The model under review builds one solid part; all positions refer to its coordinate system, in mm. A direction names the side the tool comes from. Round coordinates to 2 decimals unless told otherwise and drop trailing zeros. Order: outer loops, then holes, each group sorted by start corner. A loop starts at its lowest first (then second) coordinate and runs counter-clockwise, first axis right, second up. Notation, with made-up numbers: (-39, 2.25) -> (-30, 2.25) arc R29 cw to (-30, 37.25) -> close; hole circle Ø5 at (82.25, 25). An arc over 180 degrees is marked (long way). Use a Markdown table: item, result. Add a question column.
```python
from build123d import *

# Parameters (mm, degrees)
SKETCH1_W           = 70
SKETCH1_H           = 12
BOSS_EXTRUDE1_DEPTH = 1.5
SKETCH2_W           = 60
SKETCH2_H           = 6
CUT_EXTRUDE1_DEPTH  = 38.121422387
FILLET1_R           = 10
FILLET2_R           = 5
SKETCH3_W           = 3
SKETCH3_H           = 4
BOSS_EXTRUDE2_DEPTH = 3


with BuildPart() as part:
    # Sketch1 → Boss-Extrude1 (new, symmetric)
    with BuildSketch(Plane.XY):
        with Locations((0, 6)):
            Rectangle(SKETCH1_W, SKETCH1_H)
    extrude(amount=BOSS_EXTRUDE1_DEPTH, both=True)

    # Sketch2 → Cut-Extrude1 (cut, through all)
    with BuildSketch(Plane.XY.offset(1.5)):
        with Locations((0, 9)):
            Rectangle(SKETCH2_W, SKETCH2_H)
    extrude(amount=-CUT_EXTRUDE1_DEPTH, mode=Mode.SUBTRACT)

    # Fillet1
    # the kernel refuses this fillet: 10 mm, written as the material it adds along each edge
    with BuildSketch(Plane(origin=(30, 6, 1.5), x_dir=(-1, 0, 0), z_dir=(0, 0, -1))) as fillet1_piece_1:
        with BuildLine():
            CenterArc((9.16515139, 10), FILLET1_R, 203.578178478, 66.421821522)
            Line((0, 6), (-0.183303028, 5.92))
            ThreePointArc((-0.183303028, 5.92), (-0.2, 3), (-0.2, 0))
            Line((-0.2, 0), (0, -0.2))
            Line((0, -0.2), (9.16515139, -0.2))
            Line((9.16515139, -0.2), (9.16515139, 0))
        make_face()
    extrude(amount=3)
    with BuildSketch(Plane(origin=(-30, 6, 1.5), x_dir=(0, 1, 0), z_dir=(0, 0, -1))) as fillet1_piece_2:
        with BuildLine():
            CenterArc((10, 9.16515139), FILLET1_R, 180, 66.421821522)
            Line((0, 9.16515139), (-0.2, 9.16515139))
            Line((-0.2, 9.16515139), (-0.2, 0))
            Line((-0.2, 0), (0, -0.2))
            ThreePointArc((0, -0.2), (3, -0.2), (5.92, -0.183303028))
            Line((5.92, -0.183303028), (6, 0))
        make_face()
    extrude(amount=3)

    # Fillet2
    fillet2_edges = [part.edges().sort_by_distance(p)[0] for p in [
        (-30, 12, 0),
        (30, 12, 0),
    ]]
    fillet(fillet2_edges, radius=FILLET2_R)

    # Sketch3 → Boss-Extrude2 (add)
    with BuildSketch(Plane.XY.offset(1.5)):
        with Locations((36.5, 10)):
            Rectangle(SKETCH3_W, SKETCH3_H)
        with Locations((36.5, 2)):
            Rectangle(SKETCH3_W, SKETCH3_H)
        with Locations((-36.5, 2)):
            Rectangle(SKETCH3_W, SKETCH3_H)
        with Locations((-36.5, 10)):
            Rectangle(SKETCH3_W, SKETCH3_H)
    extrude(amount=-BOSS_EXTRUDE2_DEPTH)


solid = part.part
```
Q1. Mouldability with a two-part tool opening along Y and no side actions: class faces 1 (the flat face through (36, 8, 0)), 2 (the flat face through (-1, 0, 0)), 3 (the cylindrical face through (30.57, 11.458, -0.021)) as pulls with the +Y half, pulls with the -Y half, needs draft (parallel to the pull), parting line crosses it, or undercut.
Q2. Add section C-C (x = 12). Write out the cut boundary in (y, z).
Q3. Add section B-B (z = -0.8). Write out the cut boundary in (x, y), then the cut area to 3 significant figures.
Q4. Insertion check: pin 1 (0.9 mm diameter, centred on y = 5.5, z = 0.5, fed in from +X); pin 2 (0.9 mm diameter, centred on y = 7, z = -0.5, fed in from -X). Each pin has a flat end and moves straight along its axis. Give the tip position at first contact, or say it passes through.
Q5. Wall thickness on line 1 (Y direction, x = 0, z = -0.85); line 2 (X direction, y = 4.5, z = -0.45); line 3 (X direction, y = 11, z = -0.55): over which ranges is each line inside the solid? List them lowest first. Write a range as [from, to].
Q6. Machinability: for faces 4 (the flat face through (0, 6, 0)), 5 (the flat face through (35, 6, 0)), 6 (the flat face through (-37, 4, 0)), which of the approach directions +Z, -Z, +X, -X, +Y, -Y give a long, thin tool a straight path to every point of the face, cutting with its end or side? Answer none if there is none.
Q7. Add section A-A (y = 6.75). Write out the cut boundary in (x, z).
Q8. Add section D-D (x = -23.5). Write out the cut boundary in (y, z).
Report:
| question | item | result |
|---|---|---|
| 1 | face 1 | undercut |
| 1 | face 2 | pulls with the -Y half |
| 1 | face 3 | pulls with the +Y half |
| 2 | outline | (0, -1.5) -> (6, -1.5) -> (6, 1.5) -> (0, 1.5) -> close |
| 3 | outline | (-38, 0) -> (38, 0) -> (38, 4) -> (35, 4) -> (35, 8) -> (38, 8) -> (38, 12) -> (32.83, 12) arc R5 ccw to (28.83, 10) arc R10 cw to (20.83, 6) -> (-20.83, 6) arc R10 cw to (-28.83, 10) arc R5 ccw to (-32.83, 12) -> (-38, 12) -> (-38, 8) -> (-35, 8) -> (-35, 4) -> (-38, 4) -> close |
| 3 | area | 556 mm² |
| 4 | pin 1 | stops at x = 35 |
| 4 | pin 2 | stops at x = -35 |
| 5 | line 1 | y = [0, 6] |
| 5 | line 2 | x = [-35, 35] |
| 5 | line 3 | x = [-38, -29.83], [29.83, 38] |
| 6 | face 4 | +Z, -Z, +Y |
| 6 | face 5 | +Z, -Z, +X |
| 6 | face 6 | +Z, -Z, -X |
| 7 | outline | (-35, -1.5) -> (-24.63, -1.5) -> (-24.63, 1.5) -> (-35, 1.5) -> close; (24.63, -1.5) -> (35, -1.5) -> (35, 1.5) -> (24.63, 1.5) -> close |
| 8 | outline | (0, -1.5) -> (6.36, -1.5) -> (6.36, 1.5) -> (0, 1.5) -> close |
